Verification items for the finished model (mm, model axes). Give positions to 0.01 mm unless a question says otherwise; leave off trailing zeros. Order: outer loops, then holes, each group sorted by start corner. A loop starts at its lowest first (then second) coordinate and runs counter-clockwise, first axis right, second up.
from build123d import *

# Parameters (mm, degrees)
ESTRUSIONE_ESTRUSIONE1_DEPTH = 3
RACCORDO1_R                  = 10
SCHIZZO2_R                   = 1.75
TAGLIO_ESTRUSIONE1_DEPTH     = 3
SCHIZZO3_R                   = 1.75
TAGLIO_ESTRUSIONE2_DEPTH     = 10
SCHIZZO6_R                   = 1.6
TAGLIO_ESTRUSIONE4_DEPTH     = 10
SMUSSO1_SIZE                 = 1.5


with BuildPart() as part:
    # Schizzo1 → Estrusione-Estrusione1 (new body)
    with BuildSketch(Plane.XY):
        Polygon((172, 152), (55.74011537, 152), (-2, 94.25988463), (-2, -2), (172, -2), align=None)
    extrude(amount=ESTRUSIONE_ESTRUSIONE1_DEPTH)

    # Raccordo1
    raccordo1_edges = [part.edges().sort_by_distance(p)[0] for p in [
        (172, -2, 1.5),
        (-2, -2, 1.5),
        (-2, 94.25988463, 1.5),
        (55.74011537, 152, 1.5),
        (172, 152, 1.5),
    ]]
    fillet(raccordo1_edges, radius=RACCORDO1_R)

    # Schizzo2 → Taglio-Estrusione1 (cut)
    with BuildSketch(Plane.XY.offset(3)):
        with Locations((162, 142)):
            Circle(SCHIZZO2_R)
        with Locations((59.882250994, 142)):
            Circle(SCHIZZO2_R)
        with Locations((8, 90.117749006)):
            Circle(SCHIZZO2_R)
        with Locations((8, 8)):
            Circle(SCHIZZO2_R)
        with Locations((162, 8)):
            Circle(SCHIZZO2_R)
        with Locations((162, 73.82941029)):
            Circle(SCHIZZO2_R)
        with Locations((83.881838923, 8)):
            Circle(SCHIZZO2_R)
    extrude(amount=-TAGLIO_ESTRUSIONE1_DEPTH, mode=Mode.SUBTRACT)

    # Schizzo3 → Taglio-Estrusione2 (cut)
    with BuildSketch(Plane.XY.offset(3)):
        with Locations((151.5, 107)):
            Circle(SCHIZZO3_R)
        with Locations((30, 21)):
            Circle(SCHIZZO3_R)
    extrude(amount=-TAGLIO_ESTRUSIONE2_DEPTH, mode=Mode.SUBTRACT)

    # Schizzo6 → Taglio-Estrusione4 (cut)
    with BuildSketch(Plane.XY.offset(3)):
        with Locations((57.5, 4.5)):
            Circle(SCHIZZO6_R)
        with Locations((68.053639934, 10)):
            Circle(SCHIZZO6_R)
        with Locations((47.053639934, 10)):
            Circle(SCHIZZO6_R)
        with Locations((125.053639934, 10)):
            Circle(SCHIZZO6_R)
        with Locations((146.053639934, 10)):
            Circle(SCHIZZO6_R)
        with Locations((135.5, 4.5)):
            Circle(SCHIZZO6_R)
    extrude(amount=-TAGLIO_ESTRUSIONE4_DEPTH, mode=Mode.SUBTRACT)

    # Smusso1
    smusso1_edges = [part.edges().sort_by_distance(p)[0] for p in [
        (45.453639934, 10, 0),
        (66.453639934, 10, 0),
        (144.453639934, 10, 0),
        (55.9, 4.5, 0),
        (123.453639934, 10, 0),
        (133.9, 4.5, 0),
        (58.132250994, 142, 0),
        (6.25, 90.117749006, 0),
        (6.25, 8, 0),
        (160.25, 8, 0),
        (160.25, 73.82941029, 0),
        (82.131838923, 8, 0),
        (160.25, 142, 0),
        (149.75, 107, 0),
        (28.25, 21, 0),
    ]]
    chamfer(smusso1_edges, length=SMUSSO1_SIZE)


solid = part.part
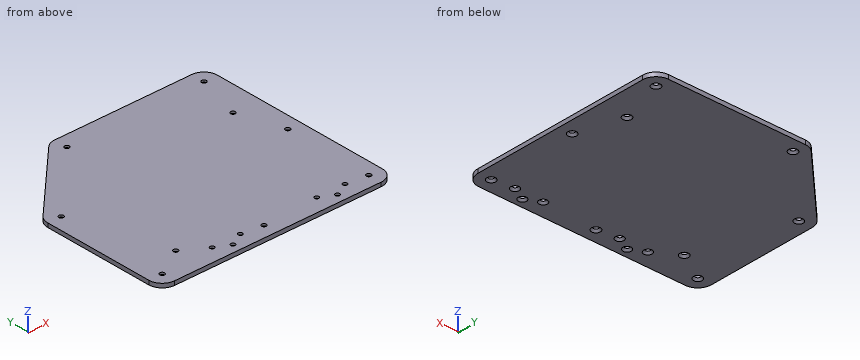
(1) Scan lines: line 1 (Y direction, x = 162, z = 2.5); line 2 (X direction, y = 90, z = 1.5); line 3 (Y direction, x = 152.5, z = 1.2). Record each from-to range of solid material in increasing order.
Solved:
line 1: y = -2 to 6.25, 9.75 to 72.08, 75.58 to 140.25, 143.75 to 152
line 2: x = -2 to 6.25, 9.75 to 172
line 3: y = -2 to 105.21, 108.79 to 152
(2) Section check A-A, the plane z = 2.2. Give the number of separate pieces and of enclosed holes in the cut face, then the cut area to 3 significant figures.
Solved:
separate pieces: 1
enclosed holes: 15
area: 24,900 mm2
(3) Section check B-B, the plane y = 126.5. Enter the section's corners in (x, z), then the cut area to 3 significant figures.
Solved:
outline: (30.24, 0) - (172, 0) - (172, 3) - (30.24, 3) - close
area: 425 mm2
(4) Go/stop test with flat-tipped pins: pin 1 (4.5 mm diameter, centred on x = 8, y = 8, fed in from -Z); pin 2 (5.5 mm diameter, centred on x = 162, y = 8, fed in from -Z); pin 3 (3.5 mm diameter, centred on x = 57.5, y = 4.5, fed in from -Z); pin 4 (4 mm diameter, centred on x = 8, y = 90.12, fed in from +Z). Record where each tip stops, or that it passes through.
Solved:
pin 1: stops at z = 1
pin 2: stops at z = 0.5
pin 3: stops at z = 1.35
pin 4: stops at z = 3
(5) Section check C-C, the plane x = 20.5. Enter the section's corners in (y, z).
Solved:
outline: (-2, 0) - (116.76, 0) - (116.76, 3) - (-2, 3) - close
